Build history of the part. All positions in model axes, mm. Face numbers are marked on the shaded views. A direction names the side the tool comes from. Coordinates: 2 decimals unless noted, no trailing zeros. Loops run counter-clockwise (first coordinate to the right, second up) from the corner with the lowest first, then second, coordinate; pieces in that order, holes last.
(1) Two-plate mould, pull along Y, no slides. Class the marked faces 3, 4, 5 and 6: pulls with the +Y half, pulls with the -Y half, needs draft (parallel to the pull), parting line crosses it, or undercut.
(2) Flat gauge pins, fed straight in: P1, Ø1.2, axis at x = 91.5, y = -139.5, coming from the -Z side; P2, Ø6, axis at x = 36.5, z = 70.5, coming from the +Y side; P3, Ø0.8, axis at x = 173.5, z = 52.5, coming from the +Y side; P4, Ø1.2, axis at y = -139.5, z = 0, coming from the -X side. Where does each tip first touch, or does it go through?
(3) Slice it at A-A (x = 69.5). Give the cut face in (y, z) (1 decimal).
(4) Slice it at D-D (z = 55). Give the cut face in (x, y).
(5) Tool access for the marked faces 1 and 2: list every direction of +Z, -Z, +X, -X, +Y, -Y with a clear straight run to the whole face (end or side of a thin tool).
(6) Wall check: L1, parallel to X at y = -56.5, z = 88.5; L2, parallel to Y at x = 21.5, z = 5.5; L3, parallel to Y at x = 124.5, z = 57. Give the ranges that are in metal, low to high.
(7) Slice it at C-C (y = -120.5). Give the cut face in (x, z).
(8) Slice it at B-B (z = 8.5). Give the cut face in (x, y), and give its area (4 significant figures).
from build123d import *

# Parameters (mm, degrees)
BOSS_EXTRUDE2_DEPTH = 174
SHELL1_START        = 1.5
SHELL1_DEPTH        = 171
SKETCH2_W           = 154
SKETCH2_H           = 5
CUT_EXTRUDE1_DEPTH  = 140


# Read off the part's stored shape, not the designer's step: Shell1
with BuildPart() as part:
    # Sketch1 → Boss-Extrude2 (new body)
    with BuildSketch(Plane.YZ):
        with BuildLine():
            Line((1.5, 20.058890221), (1.5, -1.5))
            Line((1.5, -1.5), (-140, -1.5))
            Line((-140, -1.5), (-140, 112.5))
            Line((-140, 112.5), (-75.918585959, 112.5))
            Line((-75.918585959, 112.5), (-18, 59.661991757))
            Line((-18, 59.661991757), (-18, 39.44651964))
            ThreePointArc((-18, 39.44651964), (-4.649661835, 33.373910634), (1.5, 20.058890221))
        make_face()
    extrude(amount=BOSS_EXTRUDE2_DEPTH)

    # Shell1 outline → Shell1 (cut)
    with BuildSketch(Plane.YZ.offset(SHELL1_START)):
        with BuildLine():
            ThreePointArc((0, 20), (-5.689406445, 32.292423742), (-18, 37.942407235))
            Line((-18, 37.942407235), (-18, 59.661991757))
            Line((-18, 59.661991757), (-75.918585959, 112.5))
            Line((-75.918585959, 112.5), (-138.5, 112.5))
            Line((-138.5, 112.5), (-138.5, -1.5))
            Line((-138.5, -1.5), (0, -1.5))
            Line((0, -1.5), (0, 20))
        make_face()
    extrude(amount=SHELL1_DEPTH, mode=Mode.SUBTRACT)

    # Sketch2 → Cut-Extrude1 (cut)
    with BuildSketch(Plane.XZ.offset(140)):
        with Locations((87, 1)):
            Rectangle(SKETCH2_W, SKETCH2_H)
    extrude(amount=-CUT_EXTRUDE1_DEPTH, mode=Mode.SUBTRACT)


solid = part.part
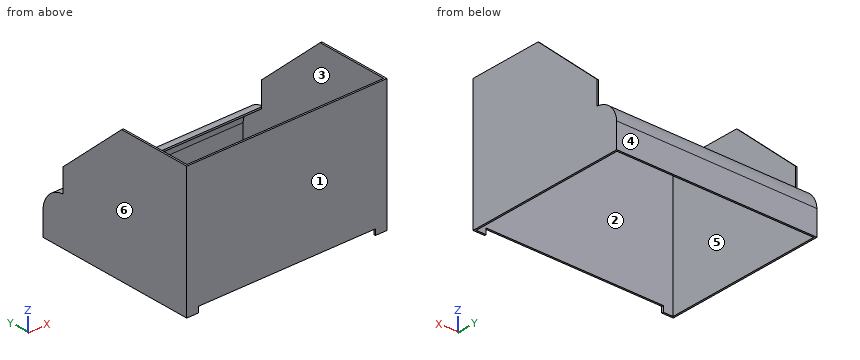
Response values:
1. face 3: undercut
1. face 4: pulls with the +Y half
1. face 5: undercut
1. face 6: needs draft
2. P1: stops at z = 3.5
2. P2: stops at y = -138.5
2. P3: stops at y = -18
2. P4: stops at x = 0
3. outline: (-140, 3.5) - (-138.5, 3.5) - (-138.5, 112.5) - (-140, 112.5) - close; (-18, 37.9) arc R19.6 cw to (0, 20) - (0, -1.5) - (1.5, -1.5) - (1.5, 20.1) arc R21.1 ccw to (-18, 39.4) - close
4. outline: (0, -140) - (174, -140) - (174, -18) - (172.5, -18) - (172.5, -138.5) - (1.5, -138.5) - (1.5, -18) - (0, -18) - close
5. face 1: +Z, -Z, +X, -X, -Y
5. face 2: +Z, -Z
6. L1: x = 0 to 1.5, 172.5 to 174
6. L2: y = -140 to -138.5, 0 to 1.5
6. L3: y = -140 to -138.5
7. outline: (0, -1.5) - (1.5, -1.5) - (1.5, 112.5) - (0, 112.5) - close; (172.5, -1.5) - (174, -1.5) - (174, 112.5) - (172.5, 112.5) - close
8. outline: (0, -140) - (174, -140) - (174, 1.5) - (0, 1.5) - close; hole (1.5, -138.5) - (172.5, -138.5) - (172.5, 0) - (1.5, 0) - close
8. area: 937.5 mm2
